Here's how the part is built. I have some questions about the finished solid (model axes, mm). Face numbers are marked on the shaded views. A direction names the side the tool comes from. Round coordinates to 2 decimals unless told otherwise and drop trailing zeros. Loops run counter-clockwise (first coordinate to the right, second up) from the corner with the lowest first, then second, coordinate; pieces in that order, holes last. Notation, with made-up numbers: M 78,76 L 107,76 A26 cw 107,102 Z; hole C 13,41.5 d10. An arc over 180 degrees is marked long. Write each question's results on one line, items separated by ' | '. Start each with the question number.
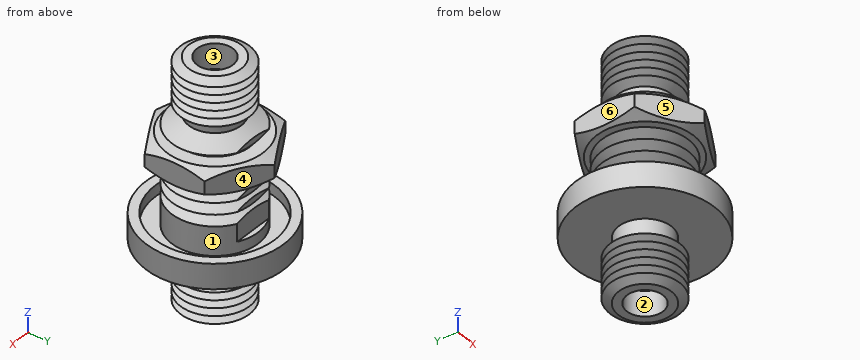
```python
from build123d import *

# Parameters (mm, degrees)
LPATTERN1_COUNT    = 5
LPATTERN1_PITCH    = 0.705555556
LPATTERN2_COUNT    = 5
LPATTERN2_PITCH    = 0.705555556
LPATTERN3_COUNT    = 6
LPATTERN3_PITCH    = 1.058333333
SKETCH5_W          = 14.29528521
SKETCH5_H          = 4.711554676
CUT_EXTRUDE1_DEPTH = 17.607404975
SKETCH7_OUTSIDE_W  = 20.78
SKETCH7_OUTSIDE_H  = 20.78
CUT_EXTRUDE2_DEPTH = 2.54


with BuildPart() as part:
    # Sketch1 → Revolve1 (revolve)
    with BuildSketch(Plane(origin=(0, 0, 0), x_dir=(0, 0, -1), z_dir=(1, 0, 0)), mode=Mode.PRIVATE) as revolve1_sk:
        Polygon((-11.684, 0), (5.842, 0), (5.842, 1.651), (8.128, 1.651), (8.128, 2.413), (7.688059095, 3.175), (4.160281317, 3.175), (3.720340412, 2.413), (2.286, 2.413), (2.286, 6.35), (0, 6.35), (0, 5.4991), (1.016, 5.4991), (1.016, 3.9751), (-7.970281317, 3.9751), (-8.872160173, 2.413), (-9.562340412, 2.413), (-10.002281317, 3.175), (-13.530059095, 3.175), (-13.97, 2.413), (-13.97, 1.651), (-11.684, 1.651), align=None)
    revolve(revolve1_sk.sketch.rotate(Axis((0, 0, -16.242320186), (0, 0, -1)), 90), axis=Axis((0, 0, -16.242320186), (0, 0, -1)))

    # Sketch2 → Cut-Revolve1 (revolve, cut)
    with BuildSketch(Plane(origin=(0, 0, 0), x_dir=(0, 0, -1), z_dir=(1, 0, 0)), mode=Mode.PRIVATE) as cut_revolve1_sk:
        Polygon((7.834706063, 3.429), (7.335281317, 2.563970965), (6.835856571, 3.429), align=None)
    cut_revolve1 = revolve(cut_revolve1_sk.sketch.rotate(Axis((0, 0, 15.0749), (0, 0, -1)), 90), axis=Axis((0, 0, 15.0749), (0, 0, -1)), mode=Mode.SUBTRACT)

    # LPattern1: Cut-Revolve1 ×5
    with Locations(*[(0, 0, i * LPATTERN1_PITCH) for i in range(1, LPATTERN1_COUNT)]):
        add(cut_revolve1, mode=Mode.SUBTRACT)

    # Sketch3 → Cut-Revolve2 (revolve, cut)
    with BuildSketch(Plane(origin=(0, 0, 0), x_dir=(0, 0, -1), z_dir=(1, 0, 0)), mode=Mode.PRIVATE) as cut_revolve2_sk:
        Polygon((-13.177281317, 2.563970965), (-12.677856571, 3.429), (-13.676706063, 3.429), align=None)
    cut_revolve2 = revolve(cut_revolve2_sk.sketch.rotate(Axis((0, 0, 15.0749), (0, 0, -1)), 90), axis=Axis((0, 0, 15.0749), (0, 0, -1)), mode=Mode.SUBTRACT)

    # LPattern2: Cut-Revolve2 ×5
    with Locations(*[(0, 0, -i * LPATTERN2_PITCH) for i in range(1, LPATTERN2_COUNT)]):
        add(cut_revolve2, mode=Mode.SUBTRACT)

    # Sketch4 → Cut-Revolve3 (revolve, cut)
    with BuildSketch(Plane(origin=(0, 0, 0), x_dir=(0, 0, -1), z_dir=(1, 0, 0)), mode=Mode.PRIVATE) as cut_revolve3_sk:
        Polygon((-7.44111465, 3.058556448), (-6.765301015, 4.2291), (-8.116928285, 4.2291), align=None)
    cut_revolve3 = revolve(cut_revolve3_sk.sketch.rotate(Axis((0, 0, 15.0749), (0, 0, -1)), 90), axis=Axis((0, 0, 15.0749), (0, 0, -1)), mode=Mode.SUBTRACT)

    # LPattern3: Cut-Revolve3 ×6
    with Locations(*[(0, 0, -i * LPATTERN3_PITCH) for i in range(1, LPATTERN3_COUNT)]):
        add(cut_revolve3, mode=Mode.SUBTRACT)

    # Sketch5 → Cut-Extrude1 (cut, through all)
    with BuildSketch(Plane.XY):
        with Locations((0, 5.860977338)):
            Rectangle(SKETCH5_W, SKETCH5_H)
    extrude(amount=CUT_EXTRUDE1_DEPTH, mode=Mode.SUBTRACT)

    # Sketch6 → Revolve2 (revolve)
    with BuildSketch(Plane(origin=(0, 0, 0), x_dir=(0, 0, -1), z_dir=(1, 0, 0)), mode=Mode.PRIVATE) as revolve2_sk:
        Polygon((-4.953, 1.294193357), (-4.953, 4.445), (-6.1468, 6.512722254), (-7.3406, 4.445), (-7.3406, 1.294193357), align=None)
    revolve(revolve2_sk.sketch.rotate(Axis((0, 0, 19.844161095), (0, 0, -1)), 331.858944442), axis=Axis((0, 0, 19.844161095), (0, 0, -1)))

    # Sketch7 outside → Cut-Extrude2 (cut)
    with BuildSketch(Plane.XY.offset(7.3406)):
        Rectangle(SKETCH7_OUTSIDE_W, SKETCH7_OUTSIDE_H)
        Polygon((0, 5.499261314), (-4.7625, 2.749630657), (-4.7625, -2.749630657), (0, -5.499261314), (4.7625, -2.749630657), (4.7625, 2.749630657), align=None, mode=Mode.SUBTRACT)
    extrude(amount=-CUT_EXTRUDE2_DEPTH, mode=Mode.SUBTRACT)


solid = part.part
```
1. I need wall thicknesses on line 1 along Y through (x, z) = (0, -0.3); line 2 along Z through (x, y) = (3.75, -2); line 3 along Z through (x, y) = (4.5, 3). Which ranges of each line are inside material? Lowest first, please.
2. I want a section at B-B on x = 3.5. Count the separate pieces of the cut face and the enclosed holes in it, plus the area to 3 significant figures.
3. I want a section at A-A on x = -5.25. List the corners of the cut face in (y, z) for me, plus the area to 3 significant figures.
4. If we mould it in two halves opening along Z, with no side actions, what happens to the marked faces 1 and 2? For each: released by +Z, released by -Z, zero draft, split by the parting line, or undercut.
5. For pin 1 (0.6 mm diameter, centred on x = -0.5, z = 3, fed in from +Y); pin 2 (3 mm diameter, centred on x = -4.5, y = -1.5, fed in from -Z); pin 3 (6 mm diameter, centred on x = 1, z = 8, fed in from +Y), each with a flat end and sliding along its axis, tell me the tip position at first contact or that it passes through.
6. Which directions (+Z, -Z, +X, -X, +Y, -Y) give clear straight access to the entire face, cutting with the end or side of a thin tool? Please do the marked faces 3, 4, 5 and 6.
Outcome:
1) line 1: -6.35 to -5.5, -3.98 to 3.98, 5.5 to 6.35 | line 2: -2.29 to -1.02, 4.95 to 7.34 | line 3: -2.29 to -1.02
2) separate pieces: 5 | enclosed holes: 0 | area: 47.7 mm2
3) outline: M -3.57,-2.29 L 3.57,-2.29 L 3.57,0 L 1.64,0 L 1.64,-1.02 L -1.64,-1.02 L -1.64,0 L -3.57,0 Z | area: 13.0 mm2
4) face 1: undercut | face 2: zero draft
5) pin 1: y = 3.51 | pin 2: z = -2.29 | pin 3: y = 5.5
6) face 3: +Z | face 4: +Z, +X, +Y | face 5: +Z, -X, -Y | face 6: +Z, -X, +Y, -Y
